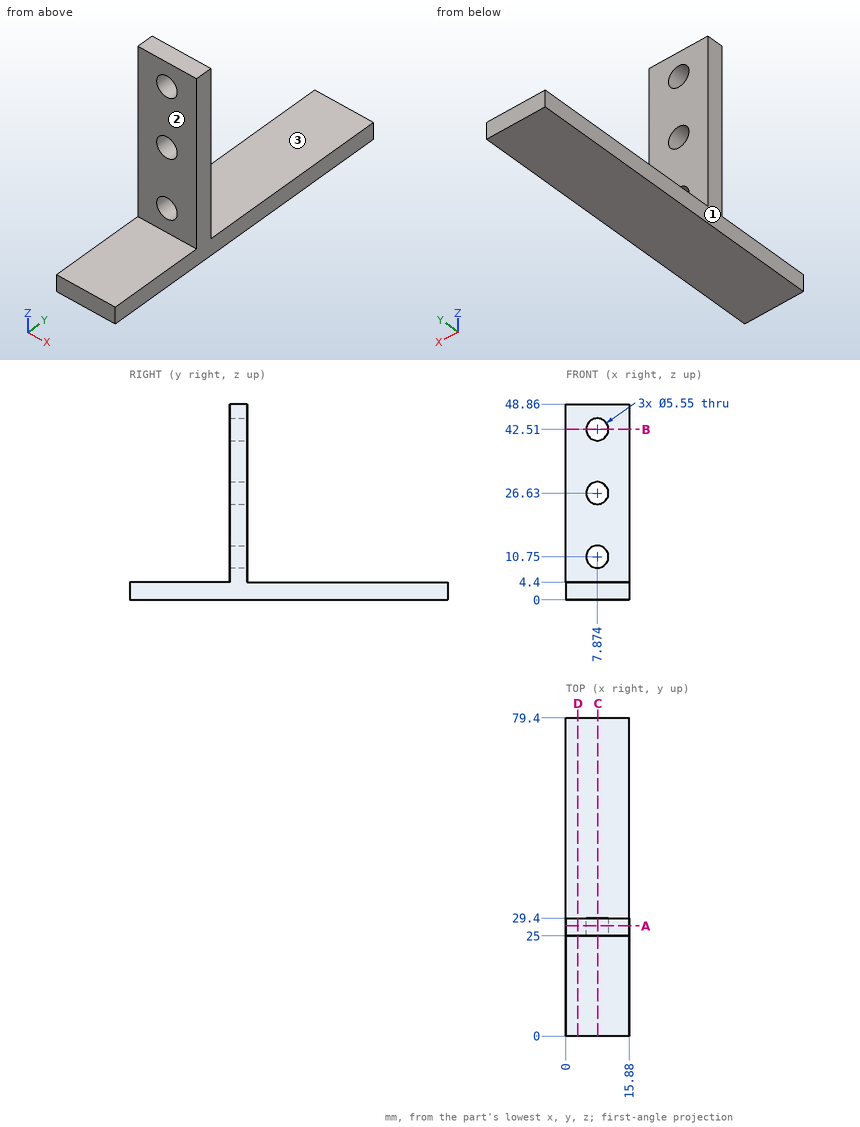
Geometry: see drawing. Coordinates: mm, zero at the bounding-box minimum. A direction names the side the tool comes from. Give positions to 0.01 mm unless a question says otherwise; leave off trailing zeros. Order: outer loops, then holes, each group sorted by start corner. A loop starts at its lowest first (then second) coordinate and runs counter-clockwise, first axis right, second up. Notation, with made-up numbers: (10, 53.5) - (48, 53.5) arc R29 ccw to (48, 89.5) - close; hole circle Ø6 at (67, 6.25). An arc over 180 degrees is marked (long way). One line per item, written item: value.
1. Cut plane A-A, the plane y = 27.5. Output: boundary loops of the cut face in (x, z) (3 decimals), and give its area (3 significant figures).
Determined:
outline: (0, 0) - (15.88, 0) - (15.88, 48.86) - (0, 48.86) - close; hole circle Ø5.55 at (7.874, 10.75); hole circle Ø5.55 at (7.874, 26.63); hole circle Ø5.55 at (7.874, 42.51)
area: 703 mm2
2. Reachability of the marked faces 1, 2 and 3 from +Z, -Z, +X, -X, +Y, -Y: full face, straight path, thin tool, end or side. Return the list, or none.
Determined:
face 1: +Z, -Z, -X, +Y, -Y
face 2: +Z, +X, -X, -Y
face 3: +Z, +X, -X, +Y
3. Cut plane D-D, the plane x = 3. Output: boundary loops of the cut face in (y, z).
Determined:
outline: (0, 0) - (79.4, 0) - (79.4, 4.4) - (29.4, 4.4) - (29.4, 48.86) - (25, 48.86) - (25, 4.4) - (0, 4.4) - close
4. Pin query (flat end, axial travel): pin 1 Ø5 at (x, y) = (10.5, 50.5) entering from +Z; pin 2 Ø2 at (y, z) = (30.5, 19.5) entering from +X; pin 3 Ø5 at (x, z) = (6, 25.5) entering from +Y; pin 4 Ø6.5 at (x, z) = (7.874, 26.63) entering from -Y. Return the tip coordinate at first contact, or that it passes through.
Determined:
pin 1: z = 4.4
pin 2: through
pin 3: y = 29.4
pin 4: y = 25
5. Cut plane B-B, the plane z = 42.51. Output: boundary loops of the cut face in (x, y), and give its area (3 significant figures).
Determined:
outline: (0, 25) - (5.1, 25) - (5.1, 29.4) - (0, 29.4) - close; (10.65, 25) - (15.88, 25) - (15.88, 29.4) - (10.65, 29.4) - close
area: 45.5 mm2
6. Cut plane C-C, the plane x = 8. Output: boundary loops of the cut face in (y, z).
Determined:
outline: (0, 0) - (79.4, 0) - (79.4, 4.4) - (29.4, 4.4) - (29.4, 7.98) - (25, 7.98) - (25, 4.4) - (0, 4.4) - close; (25, 13.52) - (29.4, 13.52) - (29.4, 23.86) - (25, 23.86) - close; (25, 29.4) - (29.4, 29.4) - (29.4, 39.74) - (25, 39.74) - close; (25, 45.28) - (29.4, 45.28) - (29.4, 48.86) - (25, 48.86) - close
7. Line query: probe 1 along Z at (x, y) = (10, 28); probe 2 along Z at (x, y) = (14.5, 17.5); probe 3 along Y at (x, z) = (15, 13.5). Output: solid intervals per line, ascending.
Determined:
probe 1: 0 to 8.97, 12.53 to 24.85, 28.41 to 40.73, 44.29 to 48.86
probe 2: 0 to 4.4
probe 3: 25 to 29.4
